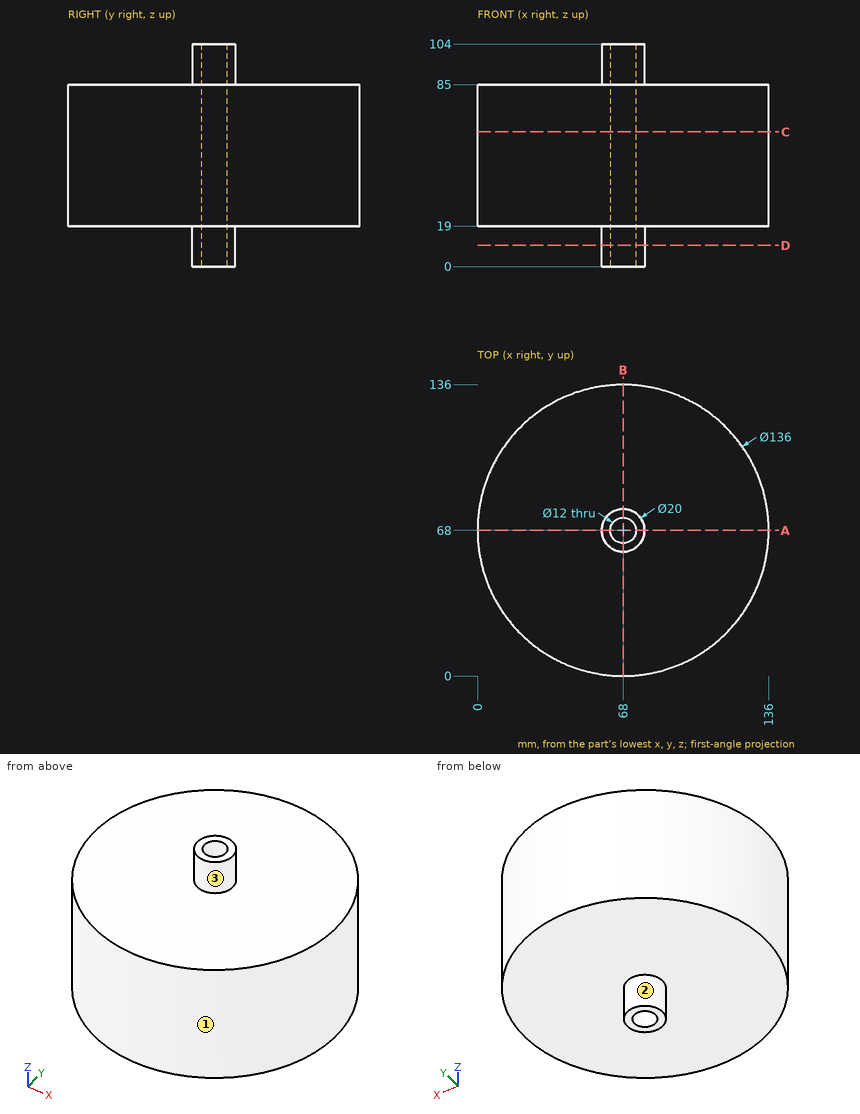
Design review of the part shown in the three views and the two pictorial views. Dimensions are in mm from the part's minimum x, y and z. A direction names the side the tool comes from. Coordinates: 2 decimals unless noted, no trailing zeros. Order: outer loops, then holes, each group sorted by start corner. A loop starts at its lowest first (then second) coordinate and runs counter-clockwise, first axis right, second up.
Item 1: For pin 1 Ø12 at (x, y) = (103.5, 45) entering from +Z; pin 2 Ø1.5 at (x, z) = (56.5, 52) entering from -Y; pin 3 Ø1 at (x, y) = (86.5, 22) entering from -Z, all flat-tipped, find the tip position at first contact; note any pin that passes through.
Item 2: For the marked faces 1, 2 and 3, list the 3-axis set-ups (+Z, -Z, +X, -X, +Y, -Y) from which the entire face can be reached by the end or side of a thin tool; tool diameter is ignored.
Item 3: Take a section at A-A, the plane y = 68. Write out the cut boundary in (x, z).
Item 4: Take a section at D-D, the plane z = 10. Write out the cut boundary in (x, y), then the cut area to 3 significant figures.
Item 5: For line 1 (Y direction, x = 68, z = 28); line 2 (X direction, y = 63, z = 94.5); line 3 (Z direction, x = 50, y = 14.5), list the stretches that pass through material, from the lowest coordinate up.
Item 6: Take a section at C-C, the plane z = 63. Write out the cut boundary in (x, y).
The answers:
1. pin 1: stops at z = 85
1. pin 2: stops at y = 0.86
1. pin 3: stops at z = 19
2. face 1: +Z, -Z
2. face 2: -Z
2. face 3: +Z
3. outline: (0, 19) - (58, 19) - (58, 0) - (62, 0) - (62, 104) - (58, 104) - (58, 85) - (0, 85) - close; (74, 0) - (78, 0) - (78, 19) - (136, 19) - (136, 85) - (78, 85) - (78, 104) - (74, 104) - close
4. outline: circle Ø20 at (68, 68); hole circle Ø12 at (68, 68)
4. area: 201 mm2
5. line 1: y = 0 to 62, 74 to 136
5. line 2: x = 59.34 to 64.68, 71.32 to 76.66
5. line 3: z = 19 to 85
6. outline: circle Ø136 at (68, 68); hole circle Ø12 at (68, 68)
